Geometry check sheet. Reference: the model listing, model coordinates, mm. A direction names the side the tool comes from. Give positions to 0.01 mm unless a question says otherwise; leave off trailing zeros. Order: outer loops, then holes, each group sorted by start corner. A loop starts at its lowest first (then second) coordinate and runs counter-clockwise, first axis right, second up. Notation, with made-up numbers: M 63.5,89.5 L 87.5,89.5 A35 ccw 87.5,125.5 Z; hole C -38.75,-28 d4. An arc over 180 degrees is marked long. Put each result on its own line as item: value. Start each with the question number.
Q1. Material ranges on L1, parallel to Y at x = -45, z = 2.4; L2, parallel to Y at x = -31, z = 0.75; L3, parallel to X at y = 7, z = 2.8, recorded low to high.
Q2. Section check A-A on y = 64.5. Record the cut outline in (x, z).
Q3. Access from +Z, -Z, +X, -X, +Y, -Y to the whole of each face (thin tool, end or side, straight path). Record for faces 1 (the flat face through (-75, 55, 2)), 2 (the flat face through (-47, 8, 2)), 3 (the flat face through (-16, 45, 5)).
Q4. Section check B-B on x = -11.45. Record the cut outline in (y, z).
Q5. Mould release check, pull along X, two halves, no side actions. Record for faces 4 (the flat face through (-25, 85, 2)), 5 (the flat face through (-40, 30.5, 2)), 6 (the flat face through (-23, 14, 2)), 7 (the flat face through (-75, 30, 2)): +X half, -X half, draft (parallel to the pull), parting line (faces both ways), or undercut.
Q6. Go/stop test with flat-tipped pins: pin 1 (7 mm diameter, centred on x = -68.55, y = 47, fed in from -Z); pin 2 (1.5 mm diameter, centred on x = -56, z = 2.5, fed in from +Y); pin 3 (1.5 mm diameter, centred on y = 62.5, z = 2.5, fed in from -X). Record where each tip stops, or that it passes through.
Q7. Section check C-C on z = 1.95. State how many separate pieces and enclosed holes the cut face has, then the cut area to 3 significant figures.
```python
from build123d import *

# Parameters (mm, degrees)
SKETCH_1_R      = 3
SKETCH_1_W      = 30
SKETCH_1_H      = 5
SKETCH_1_W_2    = 5
SKETCH_1_W_3    = 14
SKETCH_1_H_2    = 8
SKETCH_1_W_4    = 41
SKETCH_1_H_3    = 7.3
EXTRUDE_1_DEPTH = 5


with BuildPart() as part:
    # 草图1 → 凸台-拉伸1 (new body)
    with BuildSketch(Plane.XY):
        Polygon((-77.5, 0), (24.5, 0), (24.5, 26.5), (19.5, 26.5), (19.5, 56.5), (24.5, 56.5), (24.5, 83), (-25, 83), (-25, 88), (-55, 88), (-55, 83), (-77.5, 83), (-77.5, 75), (-72.5, 75), (-72.5, 55), (-77.5, 55), (-77.5, 30), (-72.5, 30), (-72.5, 10), (-77.5, 10), align=None)
        with Locations((-68.55, 47)):
            Circle(SKETCH_1_R, mode=Mode.SUBTRACT)
        with Locations((-11.45, 47)):
            Circle(SKETCH_1_R, mode=Mode.SUBTRACT)
        with BuildLine():
            Line((-57, 53), (-54, 53))
            ThreePointArc((-54, 53), (-51.171572875, 51.828427125), (-50, 49))
            Line((-50, 49), (-50, 48))
            Line((-50, 48), (-30, 48))
            Line((-30, 48), (-30, 49))
            ThreePointArc((-30, 49), (-28.828427125, 51.828427125), (-26, 53))
            Line((-26, 53), (-23, 53))
            ThreePointArc((-23, 53), (-20.878679656, 53.878679656), (-20, 56))
            Line((-20, 56), (-20, 70))
            ThreePointArc((-20, 70), (-20.878679656, 72.121320344), (-23, 73))
            Line((-23, 73), (-57, 73))
            ThreePointArc((-57, 73), (-59.121320344, 72.121320344), (-60, 70))
            Line((-60, 70), (-60, 56))
            ThreePointArc((-60, 56), (-59.121320344, 53.878679656), (-57, 53))
        make_face(mode=Mode.SUBTRACT)
        with Locations((-40, 43)):
            Rectangle(SKETCH_1_W, SKETCH_1_H, mode=Mode.SUBTRACT)
        Polygon((-55, 16), (-50, 16), (-30, 16), (-25, 16), (-25, 21), (-55, 21), align=None, mode=Mode.SUBTRACT)
        with Locations((-57.5, 11.5)):
            Rectangle(SKETCH_1_W_2, SKETCH_1_H, mode=Mode.SUBTRACT)
        with Locations((-22.5, 11.5)):
            Rectangle(SKETCH_1_W_2, SKETCH_1_H, mode=Mode.SUBTRACT)
        with Locations((-40, 8)):
            Rectangle(SKETCH_1_W_3, SKETCH_1_H_2, mode=Mode.SUBTRACT)
        with Locations((-40, 34.15)):
            Rectangle(SKETCH_1_W_4, SKETCH_1_H_3, mode=Mode.SUBTRACT)
        with Locations((-2.1, 6.27)):
            Rectangle(SKETCH_1_W_2, SKETCH_1_H_2, mode=Mode.SUBTRACT)
    extrude(amount=EXTRUDE_1_DEPTH)


solid = part.part
```
Results found:
1. L1: y = 0 to 4, 12 to 16, 21 to 30.5, 37.8 to 40.5, 45.5 to 48, 73 to 88
1. L2: y = 0 to 16, 21 to 30.5, 37.8 to 40.5, 45.5 to 48, 73 to 88
1. L3: x = -77.5 to -47, -33 to -4.6, 0.4 to 24.5
2. outline: M -72.5,0 L -60,0 L -60,5 L -72.5,5 Z; M -20,0 L 24.5,0 L 24.5,5 L -20,5 Z
3. face 1: +Z, -Z, -X
3. face 2: +Z, -Z
3. face 3: +Z, +X, -X, +Y, -Y
4. outline: M 0,0 L 44,0 L 44,5 L 0,5 Z; M 50,0 L 83,0 L 83,5 L 50,5 Z
5. face 4: +X half
5. face 5: undercut
5. face 6: undercut
5. face 7: draft
6. pin 1: stops at z = 0
6. pin 2: stops at y = 83
6. pin 3: stops at x = -72.5
7. separate pieces: 1
7. enclosed holes: 10
7. area: 6,510 mm^2
